The model under review builds one solid part; all positions refer to its coordinate system, in mm. A direction names the side the tool comes from. Round coordinates to 2 decimals unless told otherwise and drop trailing zeros. Order: outer loops, then holes, each group sorted by start corner. A loop starts at its lowest first (then second) coordinate and runs counter-clockwise, first axis right, second up.
```python
from build123d import *

# Parameters (mm, degrees)
F0_R     = 5.45
F1_DEPTH = 18
F2_E2_W  = 4
F2_E2_H  = 4
F3_DEPTH = 1.5
F4_W     = 1
F4_H     = 1
F5_DEPTH = 2.5


with BuildPart() as f1:
    # F0 (on Front) → F1 (new body)
    with BuildSketch(Plane.XZ):
        Circle(F0_R)
        with BuildLine():
            ThreePointArc((0, 3.5), (2.4748737342, 2.4748737342), (3.5, 0))
            ThreePointArc((3.5, 0), (-2.4748737342, -2.4748737342), (0, 3.5))
        make_face(mode=Mode.SUBTRACT)
    extrude(amount=F1_DEPTH)

    # F2_E2 (on explicit) → F3 (join)
    with BuildSketch(Plane(origin=(2, 0, 3.5), x_dir=(-1, 0, 0), z_dir=(0, 0, 1))):
        with Locations((2, 2)):
            Rectangle(F2_E2_W, F2_E2_H)
    extrude(amount=-F3_DEPTH)

    # F4 (on face) → F5 (cut)
    with BuildSketch(Plane(origin=(0, 0, 2), x_dir=(1, 0, 0), z_dir=(0, 0, -1))):
        with Locations((0, 2)):
            Rectangle(F4_W, F4_H)
    extrude(amount=-F5_DEPTH, mode=Mode.SUBTRACT)


solid = f1.part
```
(1) Consider section D-D (z = 4.25). Write out the cut boundary in (x, y).
Data:
outline: (-3.41, -18) - (3.41, -18) - (3.41, 0) - (-3.41, 0) - close; hole (-0.5, -2.5) - (0.5, -2.5) - (0.5, -1.5) - (-0.5, -1.5) - close
(2) Consider section B-B (x = 1.25). Write out the cut boundary in (y, z), and give its area (3 significant figures).
Data:
outline: (-18, -5.3) - (0, -5.3) - (0, -3.27) - (-18, -3.27) - close; (-18, 3.27) - (-4, 3.27) - (-4, 2) - (0, 2) - (0, 5.3) - (-18, 5.3) - close
area: 78.4 mm2
(3) Consider section C-C (y = -1). Write out the cut boundary in (x, z).
Data:
outline: circle Ø10.9 at (0, 0); hole (-2, 2) - (-2, 2.87) arc R3.5 ccw (long way) to (2, 2.87) - (2, 2) - close
(4) To check wall thickness, follow probe 1 along Z at (x, y) = (0, -3.5); probe 2 along Z at (x, y) = (1.5, -16); probe 3 along X at (y, z) = (-13, -0.5). State the ranges of each line that lie inside material, in increasing order.
Data:
probe 1: z = -5.45 to -3.5, 2 to 5.45
probe 2: z = -5.24 to -3.16, 3.16 to 5.24
probe 3: x = -5.43 to -3.46, 3.46 to 5.43
(5) Draft analysis for pull direction Y (two halves, no side actions). For faces 1 (the flat face through (0, -2, 4.5)), 2 (the flat face through (-0.1, 0, 2.5)), 3 (the flat face through (1, -2, 2)), state which applies: pulls with the +Y half, pulls with the -Y half, needs draft (parallel to the pull), parting line crosses it, or undercut.
Data:
face 1: undercut
face 2: pulls with the +Y half
face 3: needs draft
(6) Insertion check: pin 1 (1 mm diameter, centred on y = -2.5, z = 2.5, fed in from +X); pin 2 (1 mm diameter, centred on y = -2, z = 2.5, fed in from -X); pin 3 (0.8 mm diameter, centred on x = 0, z = 2.5, fed in from -Y); pin 4 (0.5 mm diameter, centred on x = 0, z = 4, fed in from +Y). Each pin has a flat end and moves straight along its axis. Give the tip position at first contact, or say it passes through.
Data:
pin 1: stops at x = 5.07
pin 2: stops at x = -5.07
pin 3: stops at y = -4
pin 4: stops at y = 0
(7) For faces 4 (the cylindrical face through (5.198, -8.874, 1.637)), 5 (the flat face through (-0.5, -2, 3)), 6 (the flat face through (0, -4, 3)), list the 3-axis set-ups (+Z, -Z, +X, -X, +Y, -Y) from which the entire face can be reached by the end or side of a thin tool; tool diameter is ignored.
Data:
face 4: +Y, -Y
face 5: none
face 6: -Y
(8) Consider section A-A (z = -3). Write out the cut boundary in (x, y), and give its area (3 significant figures).
Data:
outline: (-4.55, -18) - (-1.8, -18) - (-1.8, 0) - (-4.55, 0) - close; (1.8, -18) - (4.55, -18) - (4.55, 0) - (1.8, 0) - close
area: 98.9 mm2
